Drawing for the job (mm, zero at the part's lowest x, y, z). A direction names the side the tool comes from. Give positions to 0.01 mm unless a question says otherwise; leave off trailing zeros. Write each loop counter-clockwise with the first axis right and the second up, starting at its lowest first coordinate (ties: lowest second). Pieces come first, ordered by that corner, then holes. Notation, with made-up numbers: (82.5, 57.25) - (125.5, 57.25) arc R28 cw to (125.5, 89.25) - close; hole circle Ø5 at (41, 31). An arc over 180 degrees is marked (long way). Use CSV: the item, a comma, the result in double quotes.
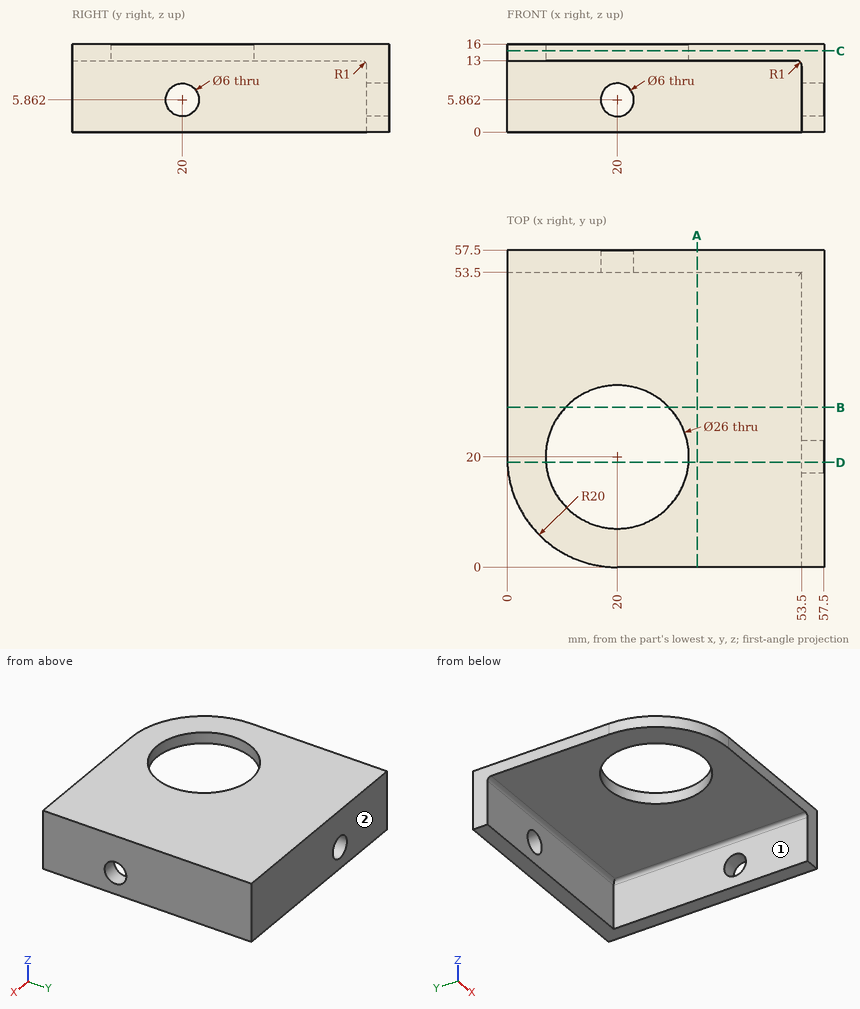
(1) Flat gauge pins, fed straight in: P1, Ø1, axis at y = 38, z = 11, coming from the -X side; P2, Ø1, axis at x = 42.5, z = 10, coming from the -Y side; P3, Ø3, axis at y = 35.5, z = 11, coming from the -X side (1 decimal); P4, Ø4, axis at x = 28.5, y = 23.5, coming from the +Z side. Where does each tip first touch, or does it go through?
Checked values:
P1,"stops at x = 53.5"
P2,"stops at y = 53.5"
P3,"stops at x = 53.4"
P4,"passes through"
(2) 3-axis set-ups, long thin cutter, end or side, ignore diameter. For the marked faces 1 and 2: which of +Z, -Z, +X, -X, +Y, -Y reach the whole face in a straight line?
Checked values:
face 1,"-Z, -X, -Y"
face 2,"+Z, -Z, +X, -X, +Y"
(3) Wall check: probe 1 along Z at (x, y) = (56.4, 20); probe 2 along Z at (x, y) = (45.5, 32); probe 3 along Y at (x, z) = (52.5, 12). Give the ranges that are in metal, low to high. Write a range as [from, to].
Checked values:
probe 1,"z = [0, 2.86], [8.86, 16]"
probe 2,"z = [13, 16]"
probe 3,"y = [53.5, 57.5]"
(4) Saw through at D-D, the plane y = 19. List the corners of the cut face in (x, z) (1 decimal).
Checked values:
outline,"(0, 13) - (7, 13) - (7, 16) - (0, 16) - close; (33, 13) - (52.5, 13) arc R1 cw to (53.5, 12) - (53.5, 8.7) - (57.5, 8.7) - (57.5, 16) - (33, 16) - close; (53.5, 0) - (57.5, 0) - (57.5, 3) - (53.5, 3) - close"
(5) Saw through at A-A, the plane x = 34.5. List the corners of the cut face in (y, z), then the cut area to 3 significant figures.
Checked values:
outline,"(0, 13) - (52.5, 13) arc R1 cw to (53.5, 12) - (53.5, 0) - (57.5, 0) - (57.5, 16) - (0, 16) - close"
area,"225 mm^2"
(6) Saw through at B-B, the plane y = 29. List the corners of the cut face in (x, z).
Checked values:
outline,"(0, 13) - (10.62, 13) - (10.62, 16) - (0, 16) - close; (29.38, 13) - (52.5, 13) arc R1 cw to (53.5, 12) - (53.5, 0) - (57.5, 0) - (57.5, 16) - (29.38, 16) - close"
(7) Saw through at C-C, the plane z = 14.75. List the corners of the cut face in (x, y).
Checked values:
outline,"(0, 20) arc R20 ccw to (20, 0) - (57.5, 0) - (57.5, 57.5) - (0, 57.5) - close; hole circle Ø26 at (20, 20)"
